```python
from build123d import *

# Parameters (mm, degrees)
SKETCH_1_W          = 129
SKETCH_1_H          = 80
EXTRUDE_1_DEPTH     = 1.6
SKETCH_2_R          = 1.575
CUT_EXTRUDE_1_DEPTH = 187.325625148
SKETCH_3_W          = 5.8
SKETCH_3_H          = 19.5
EXTRUDE_2_DEPTH     = 13.4
FILLET_1_R          = 1.5
SKETCH_4_W          = 14
SKETCH_4_H          = 9
EXTRUDE_3_DEPTH     = 11
SKETCH_5_W          = 9
SKETCH_5_H          = 11
EXTRUDE_4_DEPTH     = 0.1
CUT_EXTRUDE_2_DEPTH = 11.5
SKETCH_7_R          = 3.2
CUT_EXTRUDE_3_DEPTH = 11.5
SKETCH_8_R          = 0.75
EXTRUDE_5_DEPTH     = 10
EXTRUDE_6_DEPTH     = 14.5
SKETCH_10_W         = 6.45
SKETCH_10_H         = 5
SKETCH_10_W_2       = 6.445
CUT_EXTRUDE_4_DEPTH = 14.5
FILLET_2_R          = 1


with BuildPart() as part:
    # 草图1 → 凸台-拉伸1 (new body)
    with BuildSketch(Plane(origin=(0, 0, 0), x_dir=(1, 0, 0), z_dir=(0, 1, 0))):
        with Locations((103.769660327, 40)):
            Rectangle(SKETCH_1_W, SKETCH_1_H)
    extrude(amount=EXTRUDE_1_DEPTH)

    # 草图2 → 切除-拉伸1 (cut, through all)
    with BuildSketch(Plane(origin=(0, 1.6, 0), x_dir=(1, 0, 0), z_dir=(0, 1, 0))):
        with Locations(Location((42.269660327, 77, 0), (0, 0, 270))):
            Circle(SKETCH_2_R)
        with Locations(Location((42.269660327, 3, 0), (0, 0, 270))):
            Circle(SKETCH_2_R)
        with Locations(Location((165.269660327, 3, 0), (0, 0, 270))):
            Circle(SKETCH_2_R)
        with Locations(Location((165.269660327, 77, 0), (0, 0, 270))):
            Circle(SKETCH_2_R)
    extrude(amount=-CUT_EXTRUDE_1_DEPTH, mode=Mode.SUBTRACT)

    # 草图3 → 凸台-拉伸2 (add)
    with BuildSketch(Plane(origin=(0, 1.6, 0), x_dir=(1, 0, 0), z_dir=(0, 1, 0))):
        with Locations((158.669660327, 8.85)):
            Rectangle(SKETCH_3_W, SKETCH_3_H)
        with Locations((144.669660327, 8.85)):
            Rectangle(SKETCH_3_W, SKETCH_3_H)
        with Locations((130.669660327, 8.85)):
            Rectangle(SKETCH_3_W, SKETCH_3_H)
        with Locations((116.669660327, 8.85)):
            Rectangle(SKETCH_3_W, SKETCH_3_H)
        with Locations((102.669660327, 8.85)):
            Rectangle(SKETCH_3_W, SKETCH_3_H)
        with Locations((88.669660327, 8.85)):
            Rectangle(SKETCH_3_W, SKETCH_3_H)
        with Locations((74.669660327, 8.85)):
            Rectangle(SKETCH_3_W, SKETCH_3_H)
        with Locations((60.669660327, 8.85)):
            Rectangle(SKETCH_3_W, SKETCH_3_H)
    extrude(amount=EXTRUDE_2_DEPTH)

    # 圆角1
    fillet_1_edges = [part.edges().sort_by_distance(p)[0] for p in [
        (168.269660327, 0.8, -80),
        (168.269660327, 0.8, 0),
        (39.269660327, 0.8, 0),
        (39.269660327, 0.8, -80),
    ]]
    fillet(fillet_1_edges, radius=FILLET_1_R)

    # 草图4 → 凸台-拉伸3 (add)
    with BuildSketch(Plane(origin=(0, 1.6, 0), x_dir=(1, 0, 0), z_dir=(0, 1, 0))):
        with Locations((46.269660327, 23)):
            Rectangle(SKETCH_4_W, SKETCH_4_H)
    extrude(amount=EXTRUDE_3_DEPTH)

    # 草图5 → 凸台-拉伸4 (add)
    with BuildSketch(Plane.ZY.offset(-39.269660327)):
        with Locations((-23, 7.1)):
            Rectangle(SKETCH_5_W, SKETCH_5_H)
    extrude(amount=EXTRUDE_4_DEPTH)

    # 草图6 → 切除-拉伸2 (cut)
    with BuildSketch(Plane(origin=(53.269660327, 0, 0), x_dir=(0, 0, -1), z_dir=(1, 0, 0))):
        with BuildLine():
            Line((18.5, 12.6), (18.5, 7.6))
            ThreePointArc((18.5, 7.6), (23, 12.1), (27.5, 7.6))
            Line((27.5, 7.6), (27.5, 12.6))
            Line((27.5, 12.6), (18.5, 12.6))
        make_face()
    extrude(amount=-CUT_EXTRUDE_2_DEPTH, mode=Mode.SUBTRACT)

    # 草图7 → 切除-拉伸3 (cut)
    with BuildSketch(Plane.ZY.offset(-39.169660327)):
        with Locations((-23, 7.6)):
            Circle(SKETCH_7_R)
    extrude(amount=-CUT_EXTRUDE_3_DEPTH, mode=Mode.SUBTRACT)

    # 草图8 → 凸台-拉伸5 (add)
    with BuildSketch(Plane.ZY.offset(-50.669660327)):
        with Locations((-23, 7.6)):
            Circle(SKETCH_8_R)
    extrude(amount=EXTRUDE_5_DEPTH)

    # 草图9 → 凸台-拉伸6 (add)
    with BuildSketch(Plane(origin=(0, 1.6, 0), x_dir=(1, 0, 0), z_dir=(0, 1, 0))):
        Polygon((39.269660327, 38.3), (52.219660327, 38.3), (52.219660327, 39.565), (50.719660327, 39.565), (50.719660327, 46.015), (52.219660327, 46.015), (52.219660327, 47.285), (50.719660327, 47.285), (50.719660327, 53.73), (52.219660327, 53.73), (52.219660327, 55), (39.269660327, 55), (39.169660327, 55), (39.169660327, 53.73), (39.269660327, 53.73), (40.769660327, 53.73), (40.769660327, 47.285), (39.269660327, 47.285), (39.169660327, 47.285), (39.169660327, 46.015), (39.269660327, 46.015), (40.769660327, 46.015), (40.769660327, 39.565), (39.269660327, 39.565), (39.219660327, 39.565), (39.219660327, 38.3), align=None)
    extrude(amount=EXTRUDE_6_DEPTH)

    # 草图10 → 切除-拉伸4 (cut)
    with BuildSketch(Plane.ZY.offset(-39.219660327)):
        with Locations((-42.79, 13.6)):
            Rectangle(SKETCH_10_W, SKETCH_10_H)
        with Locations((-50.5075, 13.6)):
            Rectangle(SKETCH_10_W_2, SKETCH_10_H)
    extrude(amount=-CUT_EXTRUDE_4_DEPTH, mode=Mode.SUBTRACT)

    # 圆角2
    fillet_2_edges = [part.edges().sort_by_distance(p)[0] for p in [
        (39.169660327, 16.1, -46.65),
        (39.219660327, 16.1, -38.9325),
        (52.219660327, 16.1, -38.9325),
        (52.219660327, 16.1, -46.65),
        (52.219660327, 16.1, -54.365),
        (39.169660327, 16.1, -54.365),
    ]]
    fillet(fillet_2_edges, radius=FILLET_2_R)


solid = part.part
```
Geometry check sheet. Reference: the model listing, model coordinates, mm. A direction names the side the tool comes from. Round coordinates to 2 decimals unless told otherwise and drop trailing zeros. Loops run counter-clockwise (first coordinate to the right, second up) from the corner with the lowest first, then second, coordinate; pieces in that order, holes last. Notation, with made-up numbers: (-10.5, -37) -> (-4.5, -37) arc R17 cw to (-4.5, -32) -> close; hole circle Ø10 at (78, -6). An arc over 180 degrees is marked (long way). Use a Markdown table: item, result.
(1) Sectioned sample at B-B (z = -77). Enter the section's corners in (x, y).
Calculated:
| item | result |
|---|---|
| outline | (39.27, 0) -> (40.69, 0) -> (40.69, 1.6) -> (39.27, 1.6) -> close; (43.84, 0) -> (163.69, 0) -> (163.69, 1.6) -> (43.84, 1.6) -> close; (166.84, 0) -> (168.27, 0) -> (168.27, 1.6) -> (166.84, 1.6) -> close |
(2) Sectioned sample at A-A (x = 47.5). Enter the section's corners in (y, z) (3 decimals).
Calculated:
| item | result |
|---|---|
| outline | (0, -80) -> (1.6, -80) -> (1.6, -55) -> (16.1, -55) -> (16.1, -53.73) -> (11.1, -53.73) -> (11.1, -47.285) -> (16.1, -47.285) -> (16.1, -46.015) -> (11.1, -46.015) -> (11.1, -39.565) -> (16.1, -39.565) -> (16.1, -38.3) -> (1.6, -38.3) -> (1.6, -27.5) -> (7.6, -27.5) arc R4.5 ccw to (7.6, -18.5) -> (1.6, -18.5) -> (1.6, 0) -> (0, 0) -> close; circle Ø1.5 at (7.6, -23); hole circle Ø6.4 at (7.6, -23) |
(3) Mould release check, pull along Z, two halves, no side actions. Record for faces 6 (the flat face through (50.72, 6, -43)), 7 (the flat face through (145, 8, 0.9)), 8 (the flat face through (89, 8, -18.6)): released by +Z, released by -Z, zero draft, split by the parting line, or undercut.
Calculated:
| item | result |
|---|---|
| face 6 | undercut |
| face 7 | released by +Z |
| face 8 | released by -Z |
(4) Sectioned sample at D-D (z = -3). Give the number of separate pieces and of enclosed holes in the cut face, then the cut area to 3 significant figures.
Calculated:
| item | result |
|---|---|
| separate pieces | 3 |
| enclosed holes | 0 |
| area | 818 mm² |
(5) Go/stop test with flat-tipped pins: P1, Ø6.5, axis at y = 5, z = -12, coming from the +X side; P2, Ø2.5, axis at y = 11, z = -24, coming from the +X side; P3, Ø9, axis at x = 45.5, y = 5, coming from the +Z side. Record where each tip stops, or that it passes through.
Calculated:
| item | result |
|---|---|
| P1 | x = 161.57 |
| P2 | x = 53.27 |
| P3 | z = 0 |
(6) Scan lines: probe 1 along X at (y, z) = (1.2, -3); probe 2 along Y at (x, z) = (42, -23); probe 3 along Y at (x, z) = (41, -23). Record each from-to range of solid material in increasing order.
Calculated:
| item | result |
|---|---|
| probe 1 | 39.27 to 40.69, 43.84 to 163.69, 166.84 to 168.27 |
| probe 2 | 0 to 4.4, 6.85 to 8.35, 10.8 to 12.1 |
| probe 3 | 0 to 4.4, 6.85 to 8.35, 10.8 to 12.6 |
(7) Sectioned sample at C-C (x = 132). Enter the section's corners in (y, z), then the cut area to 3 significant figures.
Calculated:
| item | result |
|---|---|
| outline | (0, -80) -> (1.6, -80) -> (1.6, -18.6) -> (15, -18.6) -> (15, 0.9) -> (1.6, 0.9) -> (1.6, 0) -> (0, 0) -> close |
| area | 389 mm² |
(8) Set-up check for faces 1 (the flat face through (75, 15, -9)), 2 (the flat face through (147.57, 8, -9)), 3 (the cylindrical face through (41.666, 0.811, -75.545)), 4 (the flat face through (103, 8, -18.6)), 5 (the flat face through (46, 9, -38.3)): record each of +Z, -Z, +X, -X, +Y, -Y from which the full face is reachable in a straight line by a thin tool's end or side.
Calculated:
| item | result |
|---|---|
| face 1 | +Z, -Z, +X, -X, +Y |
| face 2 | +Z, -Z, +Y |
| face 3 | +Y, -Y |
| face 4 | -Z, +X, +Y |
| face 5 | +X, -X, +Y |
